Input: part model. Units: mm. Frame: model coordinates. Face numbers are marked on the shaded views. A direction names the side the tool comes from. Give positions to 0.01 mm unless a question says otherwise; leave off trailing zeros. Order: outer loops, then holes, each group sorted by start corner. A loop starts at its lowest first (then second) coordinate and runs counter-clockwise, first axis right, second up. Notation, with made-up numbers: (89.25, -18.5) - (115.25, -18.5) arc R13 cw to (115.25, -4.5) - close; hole circle Ø7 at (6, 79.25). An arc over 180 degrees is marked (long way). Answer in a Markdown table with one row per item. Add a question column.
1. Access query for the marked faces 1, 2 and 3. Directions: +Z, -Z, +X, -X, +Y, -Y. A direction counts if a zero-diameter tool reaches every point of the face in a straight line with its end or side. Return the directions, or none.
2. Section query C-C on x = 4. Return loops of the section in (y, z).
3. Contact query for flat-ended pins moving along their axis: pin 1 (11.5 mm diameter, centred on y = 9.5, z = 7.5, fed in from -X); pin 2 (20.5 mm diameter, centred on y = 2, z = -2.5, fed in from -X); pin 3 (1 mm diameter, centred on x = 7.5, y = 13, fed in from -Z); pin 4 (12 mm diameter, centred on x = -8, y = -15.5, fed in from -Z). Output: stop coordinate, or through.
4. Ray query, line 1 (Y direction, x = -8.65, z = 0); line 2 (Y direction, x = -8.8, z = 0); line 3 (X direction, y = -18, z = -3.5). Return the intervals inside material, ascending. Write a range as [from, to].
5. Section query D-D on x = -13.5. Return loops of the section in (y, z).
6. Mould query, pull axis Z, two halves, no side actions, for the marked faces 4, 5 and 6. Classes: released by +Z, released by -Z, zero draft, split by the parting line, or undercut.
```python
from build123d import *

# Parameters (mm, degrees)
BOSS_EXTRUDE1_DEPTH      = 12
BOSS_EXTRUDE1_DEPTH_BACK = 12
SKETCH1_R                = 31.75
SKETCH2_R                = 25
SKETCH2_R_2              = 16
CUT_EXTRUDE1_DEPTH       = 1
BOSS_EXTRUDE2_START      = 3
SKETCH3_R                = 16
BOSS_EXTRUDE2_DEPTH      = 3
CHAMFER2_SIZE            = 4
FILLET1_R                = 2
SKETCH4_R                = 3
BOSS_EXTRUDE3_DEPTH      = 6
SCALE1_SCALE             = 0.7761


with BuildPart() as part:
    # Sketch1 → Boss-Extrude1 (new, two sides: drawn at the far end of the back side and taken through both)
    with BuildSketch(Plane(origin=(0, 0, 0), x_dir=(0, 0, -1), z_dir=(1, 0, 0)).offset(-BOSS_EXTRUDE1_DEPTH_BACK)):
        Circle(SKETCH1_R)
    extrude(amount=BOSS_EXTRUDE1_DEPTH + BOSS_EXTRUDE1_DEPTH_BACK)

    # Sketch2 → Cut-Extrude1 (cut)
    with BuildSketch(Plane(origin=(12, 0, 0), x_dir=(0, 0, -1), z_dir=(1, 0, 0))):
        Circle(SKETCH2_R)
        Circle(SKETCH2_R_2, mode=Mode.SUBTRACT)
    cut_extrude1 = extrude(amount=-CUT_EXTRUDE1_DEPTH, mode=Mode.SUBTRACT)

    # Sketch3 → Boss-Extrude2 (add)
    with BuildSketch(Plane(origin=(12, 0, 0), x_dir=(0, 0, -1), z_dir=(1, 0, 0)).offset(BOSS_EXTRUDE2_START)):
        Circle(SKETCH3_R)
    boss_extrude2 = extrude(amount=-BOSS_EXTRUDE2_DEPTH)

    # Mirror1: Cut-Extrude1, Boss-Extrude2 across plane
    add(cut_extrude1.mirror(Plane(origin=(0, 0, 0), x_dir=(0, 0, 1), z_dir=(1, 0, 0))), mode=Mode.SUBTRACT)
    add(boss_extrude2.mirror(Plane(origin=(0, 0, 0), x_dir=(0, 0, 1), z_dir=(1, 0, 0))))

    # Chamfer2
    # the kernel refuses this chamfer: 4 mm, written as the material it takes off along each edge
    with BuildSketch(Plane(origin=(15, 0, 0), x_dir=(0, 0, -1), z_dir=(0, -1, 0))) as chamfer2_piece_1_section:
        Polygon((16, -CHAMFER2_SIZE), (16 - CHAMFER2_SIZE, 0), (16, 0), align=None)
    chamfer2_piece_1 = revolve(axis=Axis((15, 0, 0), (1, 0, 0)), mode=Mode.PRIVATE)
    chamfer2_piece_1 = split(chamfer2_piece_1, bisect_by=Plane(origin=(11, 0, 14.009360732), z_dir=(1, 0, 0)), keep=Keep.TOP, mode=Mode.PRIVATE)
    add(chamfer2_piece_1, mode=Mode.SUBTRACT)
    with BuildSketch(Plane(origin=(-15, 0, 0), x_dir=(0, 0, -1), z_dir=(0, -1, 0))) as chamfer2_piece_2_section:
        Polygon((16, CHAMFER2_SIZE), (16 - CHAMFER2_SIZE, 0), (16, 0), align=None)
    chamfer2_piece_2 = revolve(axis=Axis((-15, 0, 0), (1, 0, 0)), mode=Mode.PRIVATE)
    chamfer2_piece_2 = split(chamfer2_piece_2, bisect_by=Plane(origin=(-11, 0, 14.009360732), z_dir=(-1, 0, 0)), keep=Keep.TOP, mode=Mode.PRIVATE)
    add(chamfer2_piece_2, mode=Mode.SUBTRACT)

    # Fillet1
    fillet1_edges = [part.edges().sort_by_distance(p)[0] for p in [
        (-12, 0, 31.75),
        (12, 0, 31.75),
    ]]
    fillet(fillet1_edges, radius=FILLET1_R)

    # Sketch4 → Boss-Extrude3 (add)
    with BuildSketch(Plane(origin=(15, 0, 0), x_dir=(0, 0, -1), z_dir=(1, 0, 0))):
        Circle(SKETCH4_R)
    boss_extrude3 = extrude(amount=BOSS_EXTRUDE3_DEPTH)

    # Mirror2: Boss-Extrude3 across plane
    add(boss_extrude3.mirror(Plane(origin=(0, 0, 0), x_dir=(0, 0, 1), z_dir=(1, 0, 0))))


with BuildPart() as part_1:
    # Scale1: scaled about (0, 0, 0)
    add(part.part.scale(SCALE1_SCALE))


solid = part_1.part
```
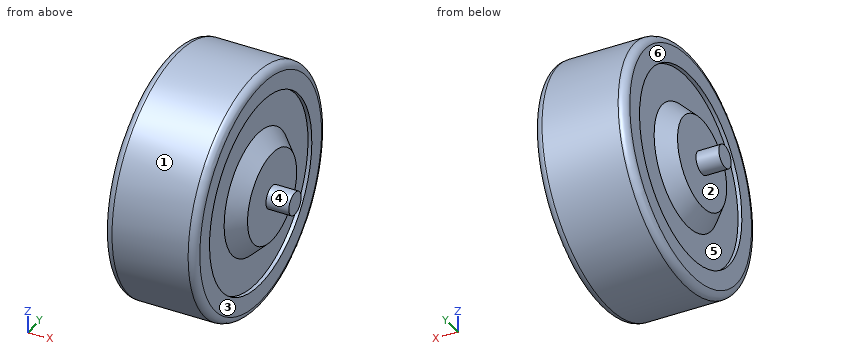
Answer:
| question | item | result |
|---|---|---|
| 1 | face 1 | +X, -X |
| 1 | face 2 | -X |
| 1 | face 3 | +X |
| 2 | outline | circle Ø49.28 at (0, 0) |
| 3 | pin 1 | stops at x = -11.64 |
| 3 | pin 2 | stops at x = -16.3 |
| 3 | pin 3 | stops at z = -21.24 |
| 3 | pin 4 | stops at z = -22.73 |
| 4 | line 1 | y = [-24.36, -19.4], [-12.3, 12.3], [19.4, 24.36] |
| 4 | line 2 | y = [-24.24, -19.4], [-12.15, 12.15], [19.4, 24.24] |
| 4 | line 3 | x = [-8.54, 8.54] |
| 5 | outline | circle Ø4.66 at (0, 0) |
| 6 | face 4 | split by the parting line |
| 6 | face 5 | undercut |
| 6 | face 6 | zero draft |
